The listing builds one solid part. Answer for the finished solid, in the listing's coordinates (mm). A direction names the side the tool comes from. Round coordinates to 2 decimals unless told otherwise and drop trailing zeros. Write each loop counter-clockwise with the first axis right and the second up, starting at its lowest first coordinate (ties: lowest second). Pieces come first, ordered by that corner, then holes. Notation, with made-up numbers: (66, -14) - (118, -14) arc R23 cw to (118, 16) - close; hole circle Ø9 at (27, 84.25). An arc over 180 degrees is marked (long way). Answer as CSV lines item,"result". Start each with the question number.
Item 1: For a pull along X with two mould halves and no side action, classify faces 1 (the flat face through (-22.54, 3.069, 10.302)), 2 (the cylindrical face through (55.88, 2.5, 0.08)), 3 (the flat face through (-9, 0, -18)), 4 (the flat face through (-28.027, 2.504, 17.066)) as pulls with the +X half, pulls with the -X half, needs draft (parallel to the pull), parting line crosses it, or undercut.
Item 2: Which of the six approach directions +Z, -Z, +X, -X, +Y, -Y give full straight-line access (tool end or side, diameter ignored) to faces 5 (the flat face through (-22.86, 1, 0)), 6 (the cylindrical face through (47.65, 8.84, 0.41)), 7 (the flat face through (28.027, 2.504, -17.066))?
Item 3: Straight lines are drawn through the part: line 1 along Y through (x, z) = (30, 11.5); line 2 along X through (y, z) = (1.25, -1.5) (1 decimal); line 3 along Z through (x, y) = (-28, 3.5). For each, find the intervals that lie inside material, in ascending order. Write a range as [from, to].
Item 4: A cutting plane is placed at D-D on y = 11. Determine the outline of the cut face in (x, z) (3 decimals).
Item 5: A cutting plane is placed at A-A on x = -12. Determine the outline of the cut face in (y, z).
Item 6: A cutting plane is placed at B-B on z = -15. Determine the outline of the cut face in (x, y), and give its area (3 significant figures).
Item 7: A cutting plane is placed at C-C on y = 1.5. Determine the outline of the cut face in (x, z), and give its area (3 significant figures).
Item 8: Flat-ended cylindrical pins translate along their axes: pin 1 (3 mm diameter, centred on y = 1.5, z = 5, fed in from +X); pin 2 (1.5 mm diameter, centred on x = 8.5, z = -16.5, fed in from -Y); pin 3 (5.5 mm diameter, centred on x = -20.5, z = 6, fed in from +Y); pin 4 (1.3 mm diameter, centred on y = 2, z = -2, fed in from -X). Find the tip coordinate at first contact, or state that the pin passes through.
```python
from build123d import *

# Parameters (mm, degrees)
SKETCH5_R             = 1.27
BOSS_EXTRUDE2_DEPTH   = 2.54
BOSS_EXTRUDE2_2_DEPTH = 2.54
BOSS_EXTRUDE1_DEPTH   = 5.08
SKETCH6_R             = 3.175
BOSS_EXTRUDE3_DEPTH   = 7.62


with BuildPart() as part:
    # Sketch5 → Boss-Extrude2 (new body)
    with BuildSketch(Plane(origin=(0, 0, 0), x_dir=(1, 0, 0), z_dir=(0, 1, 0))):
        Polygon((-22.86, 10.16), (-22.86, -10.16), (-17.78, -12.417777778), (-17.78, 12.417777778), align=None)
        with Locations(Location((-20.32, 0, 0), (0, 0, 270))):
            Circle(SKETCH5_R, mode=Mode.SUBTRACT)
    extrude(amount=BOSS_EXTRUDE2_DEPTH)



with BuildPart() as body_2:
    # Sketch5 → Boss-Extrude2 2 (new body)
    with BuildSketch(Plane(origin=(0, 0, 0), x_dir=(1, 0, 0), z_dir=(0, 1, 0))):
        Polygon((22.86, 10.16), (17.78, 12.417777778), (17.78, -12.417777778), (22.86, -10.16), align=None)
        with Locations(Location((20.32, 0, 0), (0, 0, 90))):
            Circle(SKETCH5_R, mode=Mode.SUBTRACT)
    extrude(amount=BOSS_EXTRUDE2_2_DEPTH)


with BuildPart() as part_1:
    add(part.part)

    add(body_2.part)  # Boss-Extrude1 merges body 2
    # Sketch2 → Boss-Extrude1 (add)
    with BuildSketch(Plane(origin=(0, 0, 0), x_dir=(1, 0, 0), z_dir=(0, 1, 0))):
        with BuildLine():
            Line((-53.071845065, -4.54369013), (-2.271845065, -29.94369013))
            ThreePointArc((-2.271845065, -29.94369013), (0, -30.48), (2.271845065, -29.94369013))
            Line((2.271845065, -29.94369013), (53.071845065, -4.54369013))
            ThreePointArc((53.071845065, -4.54369013), (55.88, 0), (53.071845065, 4.54369013))
            Line((53.071845065, 4.54369013), (2.271845065, 29.94369013))
            ThreePointArc((2.271845065, 29.94369013), (0, 30.48), (-2.271845065, 29.94369013))
            Line((-2.271845065, 29.94369013), (-53.071845065, 4.54369013))
            ThreePointArc((-53.071845065, 4.54369013), (-55.88, 0), (-53.071845065, -4.54369013))
        make_face()
        Polygon((-45.72, 0), (0, 20.32), (45.72, 0), (0, -20.32), align=None, mode=Mode.SUBTRACT)
    extrude(amount=BOSS_EXTRUDE1_DEPTH)

    # Sketch6 → Boss-Extrude3 (add)
    with BuildSketch(Plane(origin=(0, 5.08, 0), x_dir=(1, 0, 0), z_dir=(0, 1, 0))):
        with Locations(Location((-50.8, 0, 0), (0, 0, 90))):
            Circle(SKETCH6_R)
        with Locations(Location((50.8, 0, 0), (0, 0, 90))):
            Circle(SKETCH6_R)
    extrude(amount=BOSS_EXTRUDE3_DEPTH)


solid = part_1.part
```
Geometry says:
1,face 1,"undercut"
1,face 2,"pulls with the +X half"
1,face 3,"needs draft"
1,face 4,"pulls with the -X half"
2,face 5,"+Y, -Y"
2,face 6,"+Y"
2,face 7,"-Z, +X, +Y, -Y"
3,line 1,"y = [0, 5.08]"
3,line 2,"x = [-55.7, -42.3], [-22.9, -17.8], [17.8, 22.9], [42.3, 55.7]"
3,line 3,"z = [-17.08, -7.88], [7.88, 17.08]"
4,outline,"circle Ø6.35 at (-50.8, 0); circle Ø6.35 at (50.8, 0)"
5,outline,"(0, -25.08) - (5.08, -25.08) - (5.08, -14.99) - (0, -14.99) - close; (0, 14.99) - (5.08, 14.99) - (5.08, 25.08) - (0, 25.08) - close"
6,outline,"(-32.16, 0) - (-11.97, 0) - (-11.97, 5.08) - (-32.16, 5.08) - close; (11.97, 0) - (32.16, 0) - (32.16, 5.08) - (11.97, 5.08) - close"
6,area,"205 mm^2"
7,outline,"(-53.07, -4.54) - (-2.27, -29.94) arc R5.08 ccw to (2.27, -29.94) - (53.07, -4.54) arc R5.08 ccw to (53.07, 4.54) - (2.27, 29.94) arc R5.08 ccw to (-2.27, 29.94) - (-53.07, 4.54) arc R5.08 ccw to start; hole (-45.72, 0) - (-22.86, -10.16) - (-22.86, 10.16) - close; hole circle Ø2.54 at (-20.32, 0); hole (-17.78, -12.42) - (0, -20.32) - (17.78, -12.42) - (17.78, 12.42) - (0, 20.32) - (-17.78, 12.42) - close; hole circle Ø2.54 at (20.32, 0); hole (22.86, -10.16) - (45.72, 0) - (22.86, 10.16) - close"
7,area,"2,180 mm^2"
8,pin 1,"stops at x = 54.48"
8,pin 2,"stops at y = 0"
8,pin 3,"stops at y = 2.54"
8,pin 4,"stops at x = -55.7"
